Geometry check sheet. Reference: the model listing, model coordinates, mm. A direction names the side the tool comes from. Coordinates: 2 decimals unless noted, no trailing zeros. Order: outer loops, then holes, each group sorted by start corner. A loop starts at its lowest first (then second) coordinate and runs counter-clockwise, first axis right, second up.
```python
from build123d import *

# Parameters (mm, degrees)
SKETCH_1_R          = 1.6
EXTRUDE_1_DEPTH     = 14
SKETCH_2_W          = 6
SKETCH_2_H          = 1
CUT_EXTRUDE_1_DEPTH = 14
SKETCH_3_R          = 3.5
SKETCH_3_R_2        = 1.6
CUT_EXTRUDE_2_DEPTH = 4
EXTRUDE_2_REACH     = 32.703
SKETCH_9_W          = 7.421187745
SKETCH_9_H          = 1.2
CUT_EXTRUDE_4_DEPTH = 8


with BuildPart() as part:
    # 草图1 → 凸台-拉伸1 (new body)
    with BuildSketch(Plane.XY):
        with BuildLine():
            Line((3.354101966, 1), (27.1, 1))
            Line((27.1, 1), (27.1, -1))
            Line((27.1, -1), (3.354101966, -1))
            ThreePointArc((3.354101966, -1), (-3.5, 0), (3.354101966, 1))
        make_face()
        Circle(SKETCH_1_R, mode=Mode.SUBTRACT)
    extrude(amount=EXTRUDE_1_DEPTH)

    # 草图2 → 切除-拉伸1 (cut)
    with BuildSketch(Plane.XY.offset(14)):
        with Locations((24.1, -0.5)):
            Rectangle(SKETCH_2_W, SKETCH_2_H)
    extrude(amount=-CUT_EXTRUDE_1_DEPTH, mode=Mode.SUBTRACT)

    # 草图3 → 切除-拉伸2 (cut, symmetric)
    with BuildSketch(Plane.XY.offset(7)):
        Circle(SKETCH_3_R)
        Circle(SKETCH_3_R_2, mode=Mode.SUBTRACT)
    extrude(amount=CUT_EXTRUDE_2_DEPTH, both=True, mode=Mode.SUBTRACT)

    # 凸台-拉伸2: up to this face of the body (flat: up to its plane)
    extrude_2_end = Plane(part.part.faces().sort_by_distance((8.055556707, 0.041818565, 0))[0])
    # 草图6 → 凸台-拉伸2 (add, up to the picked face)
    with BuildSketch(Plane.XY.offset(14), mode=Mode.PRIVATE) as extrude_2_sk1:
        with BuildLine():
            Line((8.085544375, -2.1), (8.085544375, -3.4))
            Line((8.085544375, -3.4), (8.085544375, -3.5))
            Line((8.085544375, -3.5), (8.085544375, -3.728060251))
            Line((8.085544375, -3.728060251), (0, -3.728060251))
            Line((0, -3.728060251), (0, -3.5))
            ThreePointArc((0, -3.5), (2.091650066, -2.80624304), (3.354101966, -1))
            Line((3.354101966, -1), (8.085544375, -1))
            Line((8.085544375, -1), (8.085544375, -2.1))
        make_face()
    extrude_2_tool1 = split(extrude(extrude_2_sk1.sketch, amount=-EXTRUDE_2_REACH, mode=Mode.PRIVATE), bisect_by=extrude_2_end, keep=Keep.BOTH, mode=Mode.PRIVATE)
    add(extrude_2_tool1.solids().sort_by(Axis((5.088052, -2.490325, 14), (0, 0, -1)))[0])

    # 草图9 → 切除-拉伸4 (cut)
    with BuildSketch(Plane.XY.offset(11)):
        with Locations((4.374950503, -2.75)):
            Rectangle(SKETCH_9_W, SKETCH_9_H)
    extrude(amount=-CUT_EXTRUDE_4_DEPTH, mode=Mode.SUBTRACT)


solid = part.part
```
Item 1: Sectioned sample at A-A (z = 4.25). Record the cut outline in (x, y).
Item 2: Sectioned sample at B-B (z = 1.5). Record the cut outline in (x, y).
Item 3: Depth check by flat-ended pin: P1, Ø8, axis at x = 15.5, z = 11, coming from the -Y side; P2, Ø0.5, axis at y = -0.5, z = 10, coming from the +X side; P3, Ø2, axis at x = 15.5, y = 1, coming from the -Z side; P4, Ø2, axis at x = 3, z = 8, coming from the +Y side. Enter the tip coordinate at first touch or a pass-through.
Item 4: Release check for a two-part mould opening along Y. For faces 1 (the face through (1, -2, 3)), 2 (the face through (-2.87, 2, 12.48)), 3 (the face through (21.1, -0.5, 7.1)) record: pulls with the +Y half, pulls with the -Y half, needs draft (parallel to the pull), parting line crosses it, or undercut.
Item 5: Sectioned sample at C-C (y = 0.5). Record the cut outline in (x, z).
Item 6: Tool access check on faces 4 (the face through (5, -2.15, 7)), 5 (the face through (24, 0, 7)), 6 (the face through (0.505, -3.463, 7.056)), 7 (the face through (15, 1, 7)). Record the directions out of +Z, -Z, +X, -X, +Y, -Y that give a thin tool (end or side, any length) a straight path to the whole face; none if there is none.
Item 7: Sectioned sample at D-D (x = 24). Record the cut outline in (y, z).
Item 8: Thickness scan on line 1 along Z through (x, y) = (-2, 1); line 2 along Y through (x, z) = (18, 4.5); line 3 along Y through (x, z) = (24.5, 10.5). Record the ranges inside material, lowest first.
Geometry check:
1. outline: (0, -3.73) - (8.09, -3.73) - (8.09, -3.35) - (1.01, -3.35) arc R3.5 cw to (0, -3.5) - close; (2.76, -2.15) - (8.09, -2.15) - (8.09, -1) - (21.1, -1) - (21.1, 0) - (27.1, 0) - (27.1, 1) - (3.35, 1) arc R3.5 cw to start
2. outline: (0, -3.73) - (8.09, -3.73) - (8.09, -1) - (21.1, -1) - (21.1, 0) - (27.1, 0) - (27.1, 1) - (3.35, 1) arc R3.5 ccw (long way) to (0, -3.5) - close; hole circle Ø3.2 at (0, 0)
3. P1: stops at y = -1
3. P2: stops at x = 21.1
3. P3: stops at z = 0
3. P4: stops at y = 1
4. face 1: undercut
4. face 2: parting line crosses it
4. face 3: needs draft
5. outline: (-3.46, 0) - (-1.52, 0) - (-1.52, 3) - (-3.46, 3) - close; (-3.46, 11) - (-1.52, 11) - (-1.52, 14) - (-3.46, 14) - close; (1.52, 0) - (27.1, 0) - (27.1, 14) - (1.52, 14) - (1.52, 11) - (3.46, 11) - (3.46, 3) - (1.52, 3) - close
6. face 4: +X, -X
6. face 5: +Z, -Z, +X, -Y
6. face 6: -X, +Y
6. face 7: +Z, -Z, +X, +Y
7. outline: (0, 0) - (1, 0) - (1, 14) - (0, 14) - close
8. line 1: z = 0 to 3, 11 to 14
8. line 2: y = -1 to 1
8. line 3: y = 0 to 1
